Here's how the part is built. I have some questions about the finished solid (model axes, mm). Face numbers are marked on the shaded views. Round coordinates to 2 decimals unless told otherwise and drop trailing zeros. Order: outer loops, then holes, each group sorted by start corner. A loop starts at its lowest first (then second) coordinate and runs counter-clockwise, first axis right, second up. Notation, with made-up numbers: (82, -16) - (127, -16) arc R34 ccw to (127, 19) - close; hole circle Ø6 at (72, 44.5). An arc over 180 degrees is marked (long way). One line per item, written item: value.
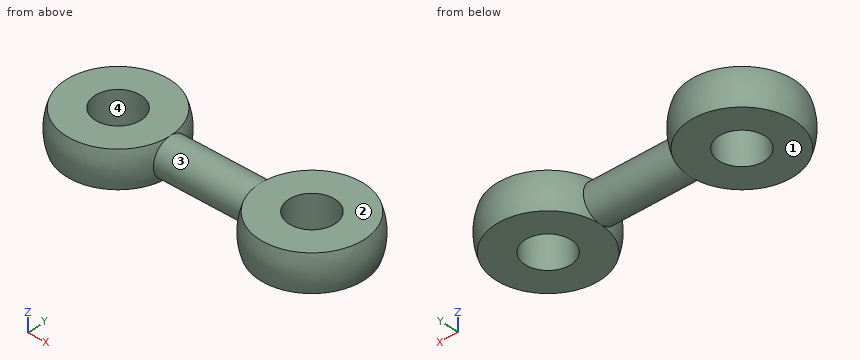
from build123d import *
from build123d.topology import SkipClean

# Parameters (mm, degrees)
CUT_EXTRUDE4_DEPTH       = 29.301943
CUT_EXTRUDE4_DEPTH_BACK  = 29.301943
CUT_EXTRUDE5_REACH       = 30.792
SKETCH5_R                = 2.5
CUT_EXTRUDE10_DEPTH      = 10
CUT_EXTRUDE10_DEPTH_BACK = 10
SKETCH9_R                = 2.5
CUT_EXTRUDE11_DEPTH      = 10


with BuildPart() as part:
    # Sketch1 → Revolve1 (revolve)
    with BuildSketch(Plane.XY, mode=Mode.PRIVATE) as revolve1_sk:
        with BuildLine():
            Line((6, 0), (-27, 0))
            ThreePointArc((-27, 0), (-22.014612, 5.913591), (-15.343146, 2))
            Line((-15.343146, 2), (-5.656854, 2))
            ThreePointArc((-5.656854, 2), (1.014612, 5.913591), (6, 0))
        make_face()
    revolve(revolve1_sk.sketch.rotate(Axis((6.214657, 0, 0), (-1, 0, 0)), 90), axis=Axis((6.214657, 0, 0), (-1, 0, 0)))

    # Sketch4 → Cut-Extrude4 (cut, two sides: drawn at the far end of the back side and taken through both)
    with SkipClean():  # the faces are left unmerged after this step: merging them gives an invalid solid
        with BuildSketch(Plane(origin=(0, 0, 0), x_dir=(1, 0, 0), z_dir=(0, 1, 0)).offset(-CUT_EXTRUDE4_DEPTH_BACK)):
            with BuildLine():
                Line((-5.656854, 2), (5.656854, 2))
                ThreePointArc((5.656854, 2), (0, 6), (-5.656854, 2))
            make_face()
            with BuildLine():
                Line((-5.656854, -2), (5.656854, -2))
                ThreePointArc((5.656854, -2), (0, -6), (-5.656854, -2))
            make_face()
        extrude(amount=CUT_EXTRUDE4_DEPTH + CUT_EXTRUDE4_DEPTH_BACK, mode=Mode.SUBTRACT)

    # Sketch5 → Cut-Extrude5 (cut, up to next)
    with BuildSketch(Plane(origin=(0, 0, -2), x_dir=(-1, 0, 0), z_dir=(0, 0, -1)), mode=Mode.PRIVATE) as cut_extrude5_sk1:
        Circle(SKETCH5_R)
    cut_extrude5_tool1 = extrude(cut_extrude5_sk1.sketch, amount=-CUT_EXTRUDE5_REACH, mode=Mode.PRIVATE) & part.part
    add(cut_extrude5_tool1.solids().sort_by_distance((0, 0, -2))[0], mode=Mode.SUBTRACT)

    # Sketch8 → Cut-Extrude10 (cut, two sides: drawn at the far end of the back side and taken through both)
    with SkipClean():  # the faces are left unmerged after this step: merging them gives an invalid solid
        with BuildSketch(Plane(origin=(0, 0, 0), x_dir=(1, 0, 0), z_dir=(0, 1, 0)).offset(-CUT_EXTRUDE10_DEPTH_BACK)):
            with BuildLine():
                Line((-15.343146, 2), (-26.656854, 2))
                ThreePointArc((-26.656854, 2), (-21, 6), (-15.343146, 2))
            make_face()
            with BuildLine():
                Line((-15.343146, -2), (-26.656854, -2))
                ThreePointArc((-26.656854, -2), (-21, -6), (-15.343146, -2))
            make_face()
        extrude(amount=CUT_EXTRUDE10_DEPTH + CUT_EXTRUDE10_DEPTH_BACK, mode=Mode.SUBTRACT)

    # Sketch9 → Cut-Extrude11 (cut)
    with SkipClean():  # the faces are left unmerged after this step: merging them gives an invalid solid
        with BuildSketch(Plane(origin=(0, 0, -2), x_dir=(-1, 0, 0), z_dir=(0, 0, -1))):
            with Locations((21, 0)):
                Circle(SKETCH9_R)
        extrude(amount=-CUT_EXTRUDE11_DEPTH, mode=Mode.SUBTRACT)


solid = part.part
Q1. Will this pin go through, and if not, where does the flat tip stop? pin 1 (1 mm diameter, centred on x = -11, z = 1.5, fed in from +Y).
Results list:
pin 1: y = 1.73
Q2. If I drill on line 1 along X through (y, z) = (0.25, 1.8); line 2 along Y through (x, z) = (-14, -0.1); line 3 along X through (y, z) = (5.25, 1.35), over which ranges is the centre line in solid material (lowest first)?
Results list:
line 1: -26.72 to -23.49, -18.51 to -2.49, 2.49 to 5.72
line 2: -2 to 2
line 3: -23.57 to -18.43, -2.57 to 2.57
Q3. We'd pull the mould along Z, two halves only. Please class the marked faces 1, 2, 3 and 4: released by +Z, released by -Z, zero draft, split by the parting line, or undercut.
Results list:
face 1: released by -Z
face 2: released by +Z
face 3: split by the parting line
face 4: zero draft
Q4. If we section it at C-C, the plane x = -10.5: Please give me the cut outline in (y, z).
Results list:
outline: circle Ø4 at (0, 0)
Q5. If we section it at A-A, the plane z = 1.6: Give the number of separate pieces and of enclosed holes in the cut face, then the cut area to 3 significant figures.
Results list:
separate pieces: 1
enclosed holes: 2
area: 194 mm²
